Could you check a few things on this model? Use its own coordinates, in mm. A direction names the side the tool comes from. Coordinates: 2 decimals unless noted, no trailing zeros. Write each loop counter-clockwise with the first axis right and the second up, starting at its lowest first coordinate (ties: lowest second). Pieces come first, ordered by that corner, then holes. Notation, with made-up numbers: M 60,-40 L 89,-40 A32 cw 89,-5 Z; hole C 13,28 d1. An arc over 180 degrees is marked long. Write item = value, one per line.
```python
from build123d import *

# Parameters (mm, degrees)
ESQUISSE1_W      = 140
ESQUISSE1_H      = 80
EXTRUSION1_DEPTH = 6
CONG_1_R         = 10
EXTRUSION2_DEPTH = 6


with BuildPart() as part:
    # Esquisse1 → Extrusion1 (new body)
    with BuildSketch(Plane.XY):
        with Locations((10, 0)):
            Rectangle(ESQUISSE1_W, ESQUISSE1_H)
    extrude(amount=EXTRUSION1_DEPTH)

    # Congé1
    cong_1_edges = [part.edges().sort_by_distance(p)[0] for p in [
        (-60, 40, 3),
        (80, 40, 3),
    ]]
    fillet(cong_1_edges, radius=CONG_1_R)

    # Esquisse6 → Extrusion2 (add)
    with BuildSketch(Plane(origin=(0, 0, 0), x_dir=(-1, 0, 0), z_dir=(0, 0, -1))):
        with BuildLine():
            Line((-50, 40), (30, 40))
            ThreePointArc((30, 40), (-10, 49.417796635), (-50, 40))
        make_face()
    extrude(amount=-EXTRUSION2_DEPTH)


solid = part.part
```
Item 1: Imagine slicing it at A-A (z = 2.65). Write out the boundary of the cut face in (x, y).
Numbers:
outline = M -60,-40 L 80,-40 L 80,30 A10 ccw 70,40 L 50,40 A89.65 ccw -30,40 L -50,40 A10 ccw -60,30 Z
Item 2: I'm going to push a flat-ended pin straight in: P1, Ø1.5, axis at y = 32.5, z = 5, coming from the -X side. Where does the tip first touch, or does it pass through?
Numbers:
P1 = -59.85
Item 3: Imagine slicing it at B-B (x = 36). Write out the boundary of the cut face in (y, z), and give its area (3 significant figures).
Numbers:
outline = M -40,0 L 45.56,0 L 45.56,6 L -40,6 Z
area = 513 mm²
Item 4: For faces 1 (the face through (60, 40, 3)), 2 (the face through (-40, 40, 3)), 3 (the face through (9, -40, 3)), which set-ups out of +Z, -Z, +X, -X, +Y, -Y let a thin tool reach every point of the face, with its end or its side?
Numbers:
face_1 = +Z, -Z, +X, +Y
face_2 = +Z, -Z, -X, +Y
face_3 = +Z, -Z, +X, -X, -Y
Item 5: Imagine slicing it at C-C (x = 57). Write out the boundary of the cut face in (y, z), and give its area (3 significant figures).
Numbers:
outline = M -40,0 L 40,0 L 40,6 L -40,6 Z
area = 480 mm²
Item 6: If I drill on line 1 along Y through (x, z) = (67.5, 2.75); line 2 along Y through (x, z) = (38.5, 1.4); line 3 along X through (y, z) = (30.5, 3.8), over which ranges is the centre line in solid material (lowest first)?
Numbers:
line_1 = -40 to 40
line_2 = -40 to 44.77
line_3 = -59.99 to 79.99
